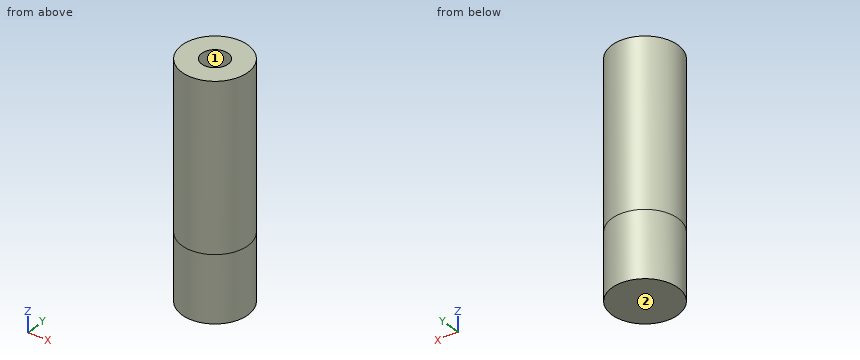
Autodesk Inventor part; units mm, degrees
ref_plane "YZ Plane" through (0, 0, 0) normal (1, 0, 0) x (0, 1, 0)
ref_plane "XZ Plane" through (0, 0, 0) normal (0, 1, 0) x (-1, 0, 0)
ref_plane "XY Plane" through (0, 0, 0) normal (0, 0, 1) x (1, 0, 0)
sketch "Sketch1" plane through (0, 0, 0) normal (0, 0, 1) x (1, 0, 0)
  circle A0 centre (0, 0) radius 10
  dimension "d0" = 20
extrude "Extrusion1" add sketch "Sketch1" along normal blind 50
sketch "Sketch2" plane through (0, 0, 50) normal (0, 0, 1) x (1, 0, 0)
  circle A0 centre (0, 0) radius 4
  dimension "d3" = 8
extrude "Extrusion2" cut sketch "Sketch2" against normal blind 15
sketch "Sketch3" plane through (0, 0, 0) normal (0, 0, -1) x (-1, 0, 0)
  point P0 (0, 0)
sketch "Sketch4" plane through (0, 0, 0) normal (0, 0, -1) x (-1, 0, 0)
  circle A0 centre (0, 0) radius 10
extrude "Extrusion3" add sketch "Sketch4" along normal blind 20
properties part number "rollers"
Geometry check sheet. Reference: the model listing, model coordinates, mm. Face numbers are marked on the shaded views. Round coordinates to 2 decimals unless told otherwise and drop trailing zeros. Order: outer loops, then holes, each group sorted by start corner. A loop starts at its lowest first (then second) coordinate and runs counter-clockwise, first axis right, second up. Notation, with made-up numbers: M 39,38.25 L 90,38.25 A22 cw 90,63.25 Z; hole C 60.5,24.25 d1. An arc over 180 degrees is marked long. Answer as CSV lines item,"result".
1) Sectioned sample at C-C on z = 2. Record the cut outline in (x, y), and give its area (3 significant figures).
Entries:
outline,"C 0,0 d20"
area,"314 mm2"
2) Sectioned sample at D-D on x = -6. Record the cut outline in (y, z).
Entries:
outline,"M -8,-20 L 8,-20 L 8,50 L -8,50 Z"
3) Mould release check, pull along Y, two halves, no side actions. Record for the marked faces 1 and 2: +Y half, -Y half, draft (parallel to the pull), parting line (faces both ways), or undercut.
Entries:
face 1,"undercut"
face 2,"draft"
4) Sectioned sample at A-A on x = 0. Record the cut outline in (y, z), and give its area (3 significant figures).
Entries:
outline,"M -10,-20 L 10,-20 L 10,50 L 4,50 L 4,35 L -4,35 L -4,50 L -10,50 Z"
area,"1,280 mm2"
5) Thickness scan on probe 1 along Y at (x, z) = (0, 40.5); probe 2 along Z at (x, y) = (-3.25, 1.75); probe 3 along Y at (x, z) = (-0.5, 18.5). Record the ranges inside material, lowest first. Write a range as [from, to].
Entries:
probe 1,"[-10, -4], [4, 10]"
probe 2,"[-20, 35]"
probe 3,"[-9.99, 9.99]"
6) Gauge pin test, flat ends, axial feed: pin 1 Ø8 at (x, z) = (-7.5, 20.5) entering from -Y; pin 2 Ø3 at (y, z) = (5, 16.5) entering from -X; pin 3 Ø1 at (x, z) = (2, 19.5) entering from -Y. Record the tip position at first contact, or that the pin passes through.
Entries:
pin 1,"y = -9.37"
pin 2,"x = -9.37"
pin 3,"y = -9.89"
